from build123d import *

# Parameters (mm, degrees)
F0_W     = 94.996
F0_H     = 77.978
F0_R     = 3
F1_DEPTH = 2
F2_W     = 64.889214
F2_H     = 53.515256
F3_DEPTH = 37
F4_R     = 9.793531
F5_DEPTH = 81


with BuildPart() as f1:
    # F0 (on Top) → F1 (new body)
    with BuildSketch(Plane.XY):
        Rectangle(F0_W, F0_H)
        with Locations((-38.5, -33)):
            Circle(F0_R, mode=Mode.SUBTRACT)
        with Locations((38.5, -33)):
            Circle(F0_R, mode=Mode.SUBTRACT)
        with Locations((-38.5, 33)):
            Circle(F0_R, mode=Mode.SUBTRACT)
        with Locations((38.5, 33)):
            Circle(F0_R, mode=Mode.SUBTRACT)
    extrude(amount=F1_DEPTH)

    # F2 (on face) → F3 (join)
    with BuildSketch(Plane(origin=(0, 0, 0), x_dir=(1, 0, 0), z_dir=(0, 0, -1))):
        Rectangle(F2_W, F2_H)
    extrude(amount=F3_DEPTH)

    # F4 (on face) → F5 (join)
    with BuildSketch(Plane.XY.offset(2)):
        Circle(F4_R)
    extrude(amount=F5_DEPTH)


solid = f1.part
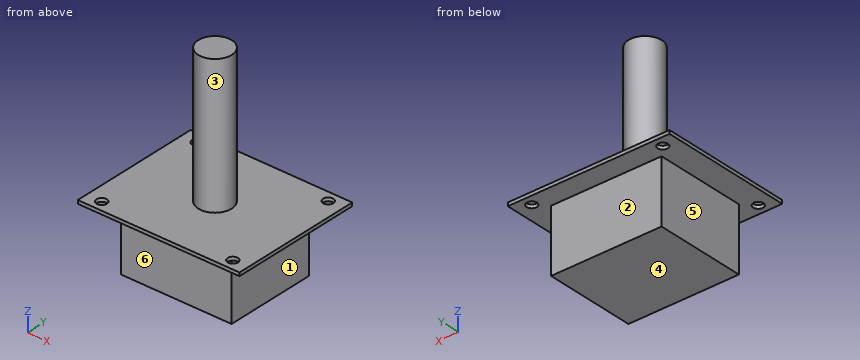
Part model, mm, in its own coordinate system. Face numbers are marked on the shaded views. A direction names the side the tool comes from. Coordinates: 2 decimals unless noted, no trailing zeros. Loops run counter-clockwise (first coordinate to the right, second up) from the corner with the lowest first, then second, coordinate; pieces in that order, holes last. Notation, with made-up numbers: (-33, 56.5) -> (-5, 56.5) arc R23 ccw to (-5, 71.5) -> close; hole circle Ø7 at (-31, 27). An arc over 180 degrees is marked (long way). Use a Markdown table: item, result. Add a question column.
Item 1: Flat gauge pins, fed straight in: P1, Ø18.5, axis at y = -0.5, z = -18.5, coming from the +X side; P2, Ø10, axis at x = 11.5, z = 59, coming from the +Y side; P3, Ø10, axis at x = -17.5, z = -9.5, coming from the +Y side. Where does each tip first touch, or does it go through?
Item 2: Probe probe 1 along Y at (x, z) = (-38.5, 0.7); probe 2 along Z at (x, y) = (2, 33); probe 3 along Z at (x, y) = (5.5, -12). List the from-to ranges inside material, lowest first.
Item 3: Band-saw the part on C-C on y = 0. Write the cut outline in (x, z).
Item 4: Band-saw the part on D-D on x = 22.5. Write the cut outline in (y, z).
Item 5: Band-saw the part on B-B on y = -33. Write the cut outline in (x, z), plus the area to 3 significant figures.
Item 6: Band-saw the part on A-A on x = 38.5. Write the cut outline in (y, z), plus the area to 3 significant figures.
Item 7: Which spindle directions (+Z, -Z, +X, -X, +Y, -Y) get a long thin tool onto all of the face, cutting with end or side? Do the marked faces 4, 5 and 6. Say none if no direction does.
Item 8: Pull direction Y, two halves, no side cores. Call the marked faces 1, 2 and 3: +Y half, -Y half, draft (parallel to the pull), parting line (faces both ways), or undercut.
Geometry says:
| question | item | result |
|---|---|---|
| 1 | P1 | x = 32.44 |
| 1 | P2 | y = 7.33 |
| 1 | P3 | y = 26.76 |
| 2 | probe 1 | -38.99 to -36, -30 to 30, 36 to 38.99 |
| 2 | probe 2 | 0 to 2 |
| 2 | probe 3 | -37 to 2 |
| 3 | outline | (-47.5, 0) -> (-32.44, 0) -> (-32.44, -37) -> (32.44, -37) -> (32.44, 0) -> (47.5, 0) -> (47.5, 2) -> (9.79, 2) -> (9.79, 83) -> (-9.79, 83) -> (-9.79, 2) -> (-47.5, 2) -> close |
| 4 | outline | (-38.99, 0) -> (-26.76, 0) -> (-26.76, -37) -> (26.76, -37) -> (26.76, 0) -> (38.99, 0) -> (38.99, 2) -> (-38.99, 2) -> close |
| 5 | outline | (-47.5, 0) -> (-41.5, 0) -> (-41.5, 2) -> (-47.5, 2) -> close; (-35.5, 0) -> (35.5, 0) -> (35.5, 2) -> (-35.5, 2) -> close; (41.5, 0) -> (47.5, 0) -> (47.5, 2) -> (41.5, 2) -> close |
| 5 | area | 166 mm² |
| 6 | outline | (-38.99, 0) -> (-36, 0) -> (-36, 2) -> (-38.99, 2) -> close; (-30, 0) -> (30, 0) -> (30, 2) -> (-30, 2) -> close; (36, 0) -> (38.99, 0) -> (38.99, 2) -> (36, 2) -> close |
| 6 | area | 132 mm² |
| 7 | face 4 | -Z, +X, -X, +Y, -Y |
| 7 | face 5 | -Z, -X, +Y, -Y |
| 7 | face 6 | -Z, +X, -X, -Y |
| 8 | face 1 | draft |
| 8 | face 2 | +Y half |
| 8 | face 3 | parting line |
